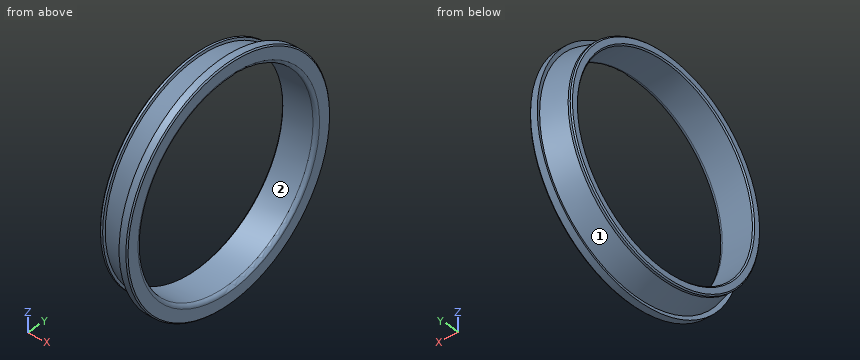
Autodesk Inventor part; units mm, degrees
ref_plane "inner_ring_XY" through (0, 0, 0) normal (0, 0, 1) x (1, 0, 0)
ref_plane "inner_ring_YZ" through (0, 0, 0) normal (1, 0, 0) x (0, 1, 0)
ref_plane "inner_ring_ZX" through (0, 0, 0) normal (0, 1, 0) x (0, 0, 1)
sketch "Sketch_1" plane through (0, 0, 0) normal (0, 0, 1) x (1, 0, 0)
  line L0 (32, 0) -> (-32, 0)
  line L1 (2, 86) -> (3, 85)
  line L2 (3, 85) -> (29, 85)
  arc A0 (29, 85) -> (32, 88) centre (29, 88) ccw
  line L3 (32, 88) -> (32, 97.75)
  line L4 (32, 97.75) -> (31, 98.75)
  line L5 (31, 98.75) -> (25.1631, 98.75)
  line L6 (25.1631, 98.75) -> (26.2196, 95.316)
  line L7 (26.2196, 95.316) -> (5.394, 89.8914)
  line L8 (5.394, 89.8914) -> (4.8095, 91.7915)
  line L9 (4.8095, 91.7915) -> (3, 91.7915)
  line L10 (3, 91.7915) -> (2, 90.7915)
  line L11 (2, 90.7915) -> (2, 86)
revolve "Revolution1" add sketch "Sketch_1" angle 360 about axis through (32, 0, 0) along (1, 0, 0)
ref_plane "inner_ring_XY" through (0, 0, 0) normal (0, 0, 1) x (1, 0, 0)
ref_plane "inner_ring_YZ" through (0, 0, 0) normal (1, 0, 0) x (0, 1, 0)
ref_plane "inner_ring_ZX" through (0, 0, 0) normal (0, 1, 0) x (0, 0, 1)
properties part number "T4DB 170_ir"
For this review, take the finished solid that the model builds, in its own axes (mm). Face numbers are marked on the shaded views. A direction names the side the tool comes from. Round coordinates to 2 decimals unless told otherwise and drop trailing zeros. Loops run counter-clockwise (first coordinate to the right, second up) from the corner with the lowest first, then second, coordinate; pieces in that order, holes last.
(1) Wall thickness on line 1 along Z through (x, y) = (22.25, 45); line 2 along Z through (x, y) = (12.5, 0); line 3 along Y through (x, z) = (26.75, -21): over which ranges is each line inside the solid? List them lowest first.
Returned:
line 1: z = -82.85 to -72.11, 72.11 to 82.85
line 2: z = -91.74 to -85, 85 to 91.74
line 3: y = -96.49 to -82.37, 82.37 to 96.49
(2) Tool access review of the marked faces 1 and 2: name each direction out of +Z, -Z, +X, -X, +Y, -Y from which nothing blocks a thin tool from reaching the whole face with its end or side.
Returned:
face 1: none
face 2: +X, -X
(3) We need section A-A (z = 0). Give the boundary of the cut face in (x, y), plus the area to 3 significant figures.
Returned:
outline: (2, -90.79) - (3, -91.79) - (4.81, -91.79) - (5.39, -89.89) - (26.22, -95.32) - (25.16, -98.75) - (31, -98.75) - (32, -97.75) - (32, -88) arc R3 ccw to (29, -85) - (3, -85) - (2, -86) - close; (2, 86) - (3, 85) - (29, 85) arc R3 ccw to (32, 88) - (32, 97.75) - (31, 98.75) - (25.16, 98.75) - (26.22, 95.32) - (5.39, 89.89) - (4.81, 91.79) - (3, 91.79) - (2, 90.79) - close
area: 517 mm2
(4) We need section C-C (x = 20). Give the boundary of the cut face in (y, z).
Returned:
outline: circle Ø187.39 at (0, 0); hole circle Ø170 at (0, 0)
(5) Clearance check with flat-ended pins moving along their axes: P1, Ø12, axis at x = 20.5, y = -44, coming from the +Z side; P2, Ø2, axis at x = 23, z = -1.5, coming from the +Y side; P3, Ø10, axis at x = 20, z = 6, coming from the -Y side. State where each tip first meets the part, or that it passes through.
Returned:
P1: stops at z = 90.19
P2: stops at y = 94.73
P3: stops at y = -94.84
